Here's how the part is built. I have some questions about the finished solid (model axes, mm). Face numbers are marked on the shaded views. Give positions to 0.01 mm unless a question says otherwise; leave off trailing zeros. Order: outer loops, then holes, each group sorted by start corner. A loop starts at its lowest first (then second) coordinate and runs counter-clockwise, first axis right, second up. Notation, with made-up numbers: M 25.5,21.25 L 48.5,21.25 A13 ccw 48.5,38.25 Z; hole C 29.5,-21 d2. An arc over 180 degrees is marked long. Use one line per item in the form item = value.
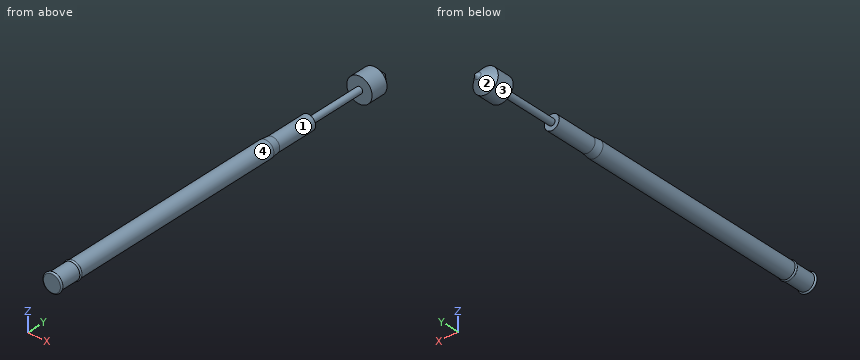
from build123d import *

# Parameters (mm, degrees)
SKETCH_1_R      = 0.835
EXTRUDE_1_DEPTH = 25
SKETCH_2_R      = 0.735
EXTRUDE_2_DEPTH = 5
SKETCH_3_R      = 0.32
EXTRUDE_3_DEPTH = 9


with BuildPart() as part:
    # 草图1 → 凸台-拉伸1 (new body)
    with BuildSketch(Plane(origin=(0, 0, 0), x_dir=(1, 0, 0), z_dir=(0, 1, 0))):
        with Locations(Location((0, 0, 0), (0, 0, 270))):
            Circle(SKETCH_1_R)
    extrude(amount=EXTRUDE_1_DEPTH)

    # 草图2 → 凸台-拉伸2 (add)
    with BuildSketch(Plane(origin=(0, 25, 0), x_dir=(1, 0, 0), z_dir=(0, 1, 0))):
        with Locations(Location((0, 0, 0), (0, 0, 270))):
            Circle(SKETCH_2_R)
    extrude(amount=EXTRUDE_2_DEPTH)

    # 草图3 → 凸台-拉伸3 (add)
    with BuildSketch(Plane(origin=(0, 30, 0), x_dir=(1, 0, 0), z_dir=(0, 1, 0))):
        with Locations(Location((0, 0, 0), (0, 0, 270))):
            Circle(SKETCH_3_R)
    extrude(amount=EXTRUDE_3_DEPTH)

    # 草图5 → 旋转1 (revolve)
    with BuildSketch(Plane.XY, mode=Mode.PRIVATE) as revolve_1_sk:
        Polygon((0.835, 25), (0.735, 25.8), (0.735, 25), align=None)
        with BuildLine():
            Line((0.835, 0.23), (0.835, 0))
            ThreePointArc((0.835, 0), (0.95, 0.115), (0.835, 0.23))
        make_face()
        with BuildLine():
            Line((0.835, 2.5), (0.835, 2.27))
            ThreePointArc((0.835, 2.27), (0.915, 2.385), (0.835, 2.5))
        make_face()
    revolve(revolve_1_sk.sketch.rotate(Axis((0, 0, 0), (0, 1, 0)), 90), axis=Axis((0, 0, 0), (0, 1, 0)))

    # 草图6 → 旋转2 (revolve)
    with BuildSketch(Plane.XY, mode=Mode.PRIVATE) as revolve_2_sk:
        Polygon((0, 39), (-1.25, 37.75), (-1.25, 36), (0, 36), align=None)
    revolve(revolve_2_sk.sketch.rotate(Axis((0, 0, 0), (0, -1, 0)), 90), axis=Axis((0, 0, 0), (0, -1, 0)))

    # 草图7 → 切除-旋转5 (revolve, cut)
    with BuildSketch(Plane.XY, mode=Mode.PRIVATE) as cut_revolve_5_sk:
        Polygon((0.32, 39), (0.02, 39), (0.32, 38.68), align=None)
    revolve(cut_revolve_5_sk.sketch.rotate(Axis((0, 0, 0), (0, -1, 0)), 270), axis=Axis((0, 0, 0), (0, -1, 0)), mode=Mode.SUBTRACT)


solid = part.part
Q1. I need wall thicknesses on L1, parallel to Y at x = 0.85, z = -0.2; L2, parallel to Y at x = 0.5, z = -0.35; L3, parallel to Y at x = 0.5, z = -0.45. Which ranges of each line are inside material? Lowest first, please.
Found:
L1 = 0.01 to 0.22, 2.29 to 2.48, 36 to 38.13
L2 = 0 to 30, 36 to 38.39
L3 = 0 to 30, 36 to 38.33
Q2. I want a section at A-A on y = 22. Write out the boundary of the cut face in (x, z) (3 decimals).
Found:
outline = C 0,0 d1.67
Q3. I'm going to push flat-ended pins straight in: pin 1 Ø0.7 at (x, z) = (-0.5, 0) entering from +Y; pin 2 Ø1.5 at (x, z) = (0, 1) entering from +Y. Where does each tip first touch, or does it pass through?
Found:
pin_1 = 38.86
pin_2 = 38.75
Q4. I want a section at B-B on y = 32.5. Write out the boundary of the cut face in (x, z), then the cut area to 3 significant figures.
Found:
outline = C 0,0 d0.64
area = 0.322 mm²
Q5. Thinking about a two-plate mould opening in Y: for the marked faces 1, 2, 3 and 4, which applies, +Y half, -Y half, draft (parallel to the pull), parting line (faces both ways), or undercut?
Found:
face_1 = undercut
face_2 = +Y half
face_3 = draft
face_4 = undercut
